Model file for the job. Use its own axes, mm. Face numbers are marked on the shaded views. A direction names the side the tool comes from. Give positions to 0.01 mm unless a question says otherwise; leave off trailing zeros. Write each loop counter-clockwise with the first axis right and the second up, starting at its lowest first coordinate (ties: lowest second). Pieces come first, ordered by that corner, then holes. Notation, with made-up numbers: (24.25, -14.75) - (45.25, -14.75) arc R29 ccw to (45.25, 22.25) - close; hole circle Ø1 at (11.25, -27). An arc over 180 degrees is marked (long way). One line per item, written item: value. Start each with the question number.
(1) Cut at B-B, the plane z = 0. List the corners of the cut face in (x, y), and give its area (3 significant figures).
(2) Mould opens along X. For the marked faces 3 and 4 say: pulls with the +X half, pulls with the -X half, needs draft (parallel to the pull), parting line crosses it, or undercut.
(3) Cut at D-D, the plane z = -55. List the corners of the cut face in (x, y), and give its area (3 significant figures).
(4) 3-axis set-ups, long thin cutter, end or side, ignore diameter. For the marked faces 1 and 2: which of +Z, -Z, +X, -X, +Y, -Y reach the whole face in a straight line?
(5) Cut at A-A, the plane x = 0. List the corners of the cut face in (y, z), and give its area (3 significant figures).
(6) Probe L1, parallel to Z at x = 0, y = 10; L2, parallel to Y at x = 16, z = -59; L3, parallel to X at y = 12, z = -7.5. List the from-to ranges inside material, lowest first.
(7) Drop flat-ended pins along their axis: P1, Ø8, axis at y = 18, z = 18.5, coming from the +X side; P2, Ø12.5, axis at x = -29, z = 79.5, coming from the +Y side; P3, Ø5, axis at x = -48, y = 11, coming from the +Z side. Give the stop position or say it passes through.
(8) Cut at C-C, the plane y = 20. List the corners of the cut face in (x, z).
from build123d import *

# Parameters (mm, degrees)
SKETCH1_R           = 70
BOSS_EXTRUDE1_DEPTH = 33
SKETCH4_W           = 36
SKETCH4_H           = 33.003390547
BOSS_EXTRUDE2_DEPTH = 8
BOSS_EXTRUDE3_DEPTH = 23
SKETCH10_R          = 13.35
CUT_EXTRUDE1_DEPTH  = 14
CHAMFER2_SIZE       = 6


with BuildPart() as part:
    # Sketch1 → Boss-Extrude1 (new body)
    with BuildSketch(Plane(origin=(0, 0, 0), x_dir=(1, 0, 0), z_dir=(0, 1, 0))):
        Circle(SKETCH1_R)
    extrude(amount=BOSS_EXTRUDE1_DEPTH)

    # Sketch4 → Boss-Extrude2 (add)
    with BuildSketch(Plane(origin=(-21.221579415, 0, 64.231180646), x_dir=(0.949517333, 0, 0.313714574), z_dir=(-0.313714574, 0, 0.949517333))):
        with Locations((0, 16.501695274)):
            Rectangle(SKETCH4_W, SKETCH4_H)
    extrude(amount=BOSS_EXTRUDE2_DEPTH)

    # Sketch7 → Boss-Extrude3 (add)
    with BuildSketch(Plane(origin=(-23.731296009, 0, 71.827319311), x_dir=(0.949517333, 0, 0.313714574), z_dir=(-0.313714574, 0, 0.949517333))):
        with BuildLine():
            Line((-9.5, 26.2), (9.5, 26.2))
            ThreePointArc((9.5, 26.2), (14.25, 21.45), (9.5, 16.7))
            Line((9.5, 16.7), (-9.5, 16.7))
            ThreePointArc((-9.5, 16.7), (-14.25, 21.45), (-9.5, 26.2))
        make_face()
    extrude(amount=BOSS_EXTRUDE3_DEPTH)

    # Sketch10 → Cut-Extrude1 (cut)
    with BuildSketch(Plane.XZ):
        Circle(SKETCH10_R)
    extrude(amount=-CUT_EXTRUDE1_DEPTH, mode=Mode.SUBTRACT)

    # Chamfer2
    chamfer2_edges = [part.edges().sort_by_distance(p)[0] for p in [
        (-13.35, 0, 0),
    ]]
    chamfer(chamfer2_edges, length=CHAMFER2_SIZE)


solid = part.part
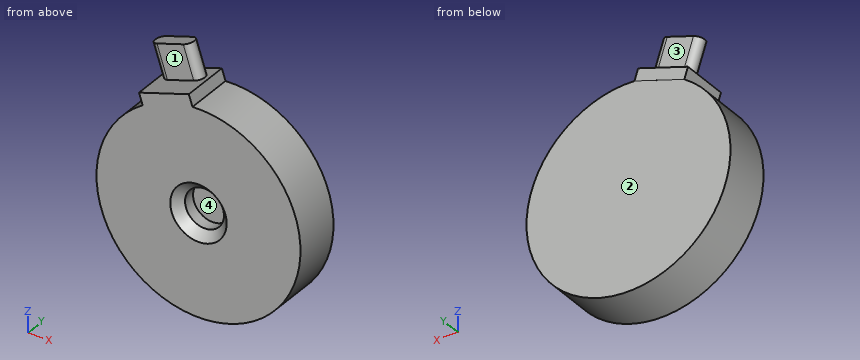
Answers follow:
1. outline: (-70, 0) - (-19.35, 0) - (-13.35, 6) - (-13.35, 14) - (13.35, 14) - (13.35, 6) - (19.35, 0) - (70, 0) - (70, 33) - (-70, 33) - close
1. area: 4,210 mm²
2. face 3: needs draft
2. face 4: undercut
3. outline: (-43.3, 0) - (43.3, 0) - (43.3, 33) - (-43.3, 33) - close
3. area: 2,860 mm²
4. face 1: +Z, -X, -Y
4. face 2: +Z, -Z, +X, -X, +Y
5. outline: (0, -70) - (33, -70) - (33, 70) - (0, 70) - (0, 19.35) - (6, 13.35) - (14, 13.35) - (14, -13.35) - (6, -13.35) - (0, -19.35) - close
5. area: 4,210 mm²
6. L1: z = -70 to -13.35, 13.35 to 70
6. L2: y = 0 to 33
6. L3: x = -69.6 to -11.04, 11.04 to 69.6
7. P1: stops at x = 68.48
7. P2: stops at y = 26.2
7. P3: stops at z = 53.2
8. outline: (-44.26, 89.27) - (-37.05, 67.43) - (-40.82, 66.18) - (-38.31, 58.58) arc R70 ccw (long way) to (-4.13, 69.88) - (-6.64, 77.47) - (-10.42, 76.23) - (-17.63, 98.07) - close
